Can you work these out from the drawing? Everything is in mm from the part's minimum corner. A direction names the side the tool comes from. Coordinates: 2 decimals unless noted, no trailing zeros. Write each loop counter-clockwise with the first axis right and the second up, starting at its lowest first coordinate (ties: lowest second). Pieces come first, ordered by that corner, then holes.
(1) For pin 1 Ø1.6 at (y, z) = (2, 12) entering from -X; pin 2 Ø1.5 at (y, z) = (2, 11.5) entering from +X; pin 3 Ø0.6 at (x, y) = (7, 3.5) entering from +Z (1 decimal); pin 4 Ø1.5 at (x, y) = (11.5, 5.5) entering from -Z, each with a flat end and sliding along its axis, tell me the tip position at first contact or that it passes through.
(2) Imagine slicing it at C-C, the plane z = 12. List the corners of the cut face in (x, y) for me (1 decimal).
(3) Which directions (+Z, -Z, +X, -X, +Y, -Y) give clear straight access to the entire face, cutting with the end or side of a thin tool? Please do the marked faces 1, 2, 3 and 4.
(4) Imagine slicing it at B-B, the plane y = 3.25. List the corners of the cut face in (x, z) for me (1 decimal).
(5) Please list where these lines run through material, in increasing order: probe 1 along Y at (x, z) = (1, 3.75); probe 2 along Z at (x, y) = (12.25, 0.5).
(6) Imagine slicing it at A-A, the plane y = 1.5. List the corners of the cut face in (x, z) for me (1 decimal).
(7) Imagine slicing it at D-D, the plane x = 4.5. List the corners of the cut face in (y, z) for me.
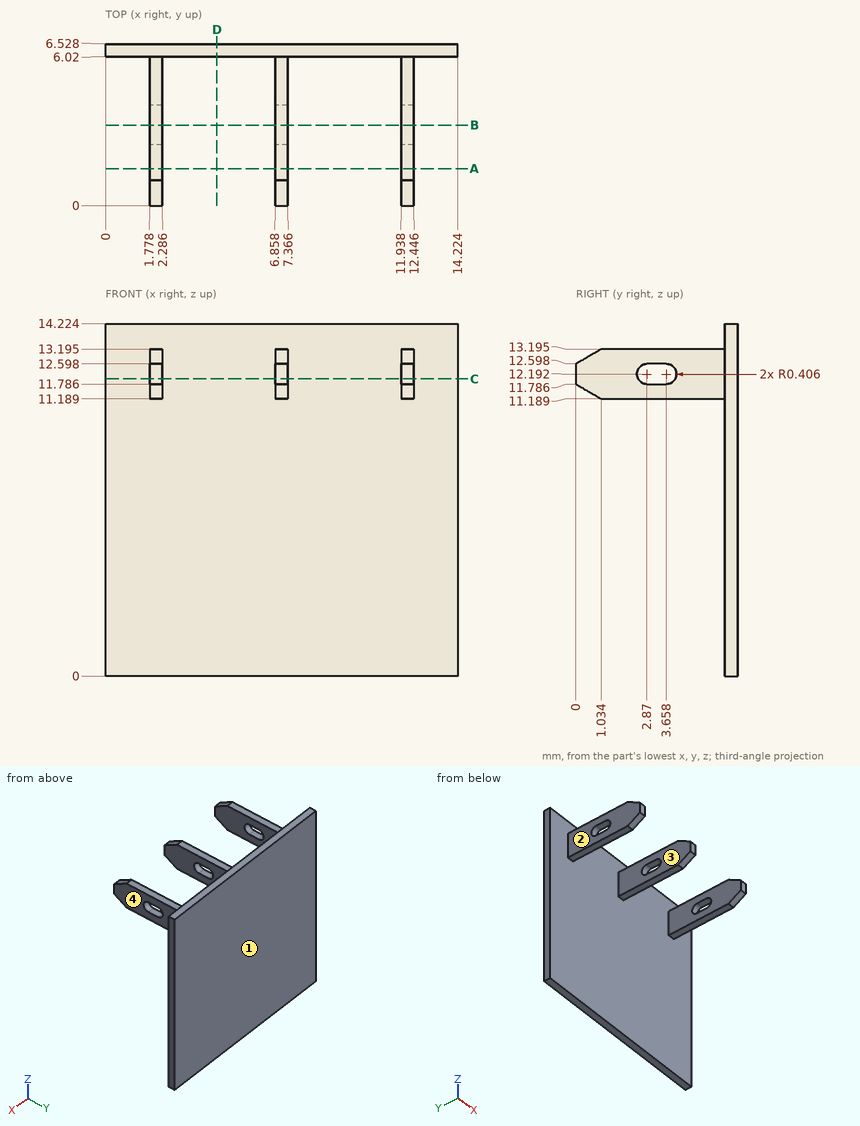
Recorded:
1. pin 1: stops at x = 1.78
1. pin 2: stops at x = 12.45
1. pin 3: stops at z = 13.2
1. pin 4: stops at z = 0
2. outline: (0, 6) - (1.8, 6) - (1.8, 4) - (2.3, 4) - (2.3, 6) - (6.9, 6) - (6.9, 4) - (7.4, 4) - (7.4, 6) - (11.9, 6) - (11.9, 4) - (12.4, 4) - (12.4, 6) - (14.2, 6) - (14.2, 6.5) - (0, 6.5) - close; (1.8, 0) - (2.3, 0) - (2.3, 2.5) - (1.8, 2.5) - close; (6.9, 0) - (7.4, 0) - (7.4, 2.5) - (6.9, 2.5) - close; (11.9, 0) - (12.4, 0) - (12.4, 2.5) - (11.9, 2.5) - close
3. face 1: +Z, -Z, +X, -X, +Y
3. face 2: +Z, -Z, -X, -Y
3. face 3: +Z, -Z, -Y
3. face 4: +Z, -Z, +X, -Y
4. outline: (1.8, 11.2) - (2.3, 11.2) - (2.3, 11.8) - (1.8, 11.8) - close; (1.8, 12.6) - (2.3, 12.6) - (2.3, 13.2) - (1.8, 13.2) - close; (6.9, 11.2) - (7.4, 11.2) - (7.4, 11.8) - (6.9, 11.8) - close; (6.9, 12.6) - (7.4, 12.6) - (7.4, 13.2) - (6.9, 13.2) - close; (11.9, 11.2) - (12.4, 11.2) - (12.4, 11.8) - (11.9, 11.8) - close; (11.9, 12.6) - (12.4, 12.6) - (12.4, 13.2) - (11.9, 13.2) - close
5. probe 1: y = 6.02 to 6.53
5. probe 2: z = 11.5 to 12.89
6. outline: (1.8, 11.2) - (2.3, 11.2) - (2.3, 13.2) - (1.8, 13.2) - close; (6.9, 11.2) - (7.4, 11.2) - (7.4, 13.2) - (6.9, 13.2) - close; (11.9, 11.2) - (12.4, 11.2) - (12.4, 13.2) - (11.9, 13.2) - close
7. outline: (6.02, 0) - (6.53, 0) - (6.53, 14.22) - (6.02, 14.22) - close
